```python
from build123d import *

# Parameters (mm, degrees)
SKETCH_1_W      = 20
SKETCH_1_H      = 13.2
SKETCH_1_R      = 1
EXTRUDE_1_DEPTH = 1.3
SKETCH_1_3_W    = 3.8
SKETCH_1_3_H    = 4.7
EXTRUDE_2_DEPTH = 3
SKETCH_1_4_W    = 1.6
SKETCH_1_4_H    = 0.7
EXTRUDE_3_DEPTH = 2.2
SKETCH_1_5_W    = 3.5
SKETCH_1_5_H    = 3
EXTRUDE_4_DEPTH = 3.5


with BuildPart() as part:
    # Sketch 1 → Extrude 1 (new body)
    with BuildSketch(Plane(origin=(0, 0, 0), x_dir=(1, 0, 0), z_dir=(0, 1, 0))):
        Rectangle(SKETCH_1_W, SKETCH_1_H)
        with Locations(Location((8.6, 5.2, 0), (0, 0, 270))):
            Circle(SKETCH_1_R, mode=Mode.SUBTRACT)
        with Locations(Location((-8.6, -5.2, 0), (0, 0, 270))):
            Circle(SKETCH_1_R, mode=Mode.SUBTRACT)
    extrude(amount=EXTRUDE_1_DEPTH)

    # Sketch 1_3 → Extrude 2 (add)
    with BuildSketch(Plane(origin=(0, 0, 0), x_dir=(1, 0, 0), z_dir=(0, 1, 0))):
        with Locations((-3.1, 3.25)):
            Rectangle(SKETCH_1_3_W, SKETCH_1_3_H)
        with Locations((-3.1, -3.25)):
            Rectangle(SKETCH_1_3_W, SKETCH_1_3_H)
    extrude(amount=EXTRUDE_2_DEPTH)

    # Sketch 1_4 → Extrude 3 (add)
    with BuildSketch(Plane(origin=(0, 0, 0), x_dir=(1, 0, 0), z_dir=(0, 1, 0))):
        with Locations((3.1, 4.65)):
            Rectangle(SKETCH_1_4_W, SKETCH_1_4_H)
        with Locations((3.1, 2.45)):
            Rectangle(SKETCH_1_4_W, SKETCH_1_4_H)
        with Locations((3.1, 0.25)):
            Rectangle(SKETCH_1_4_W, SKETCH_1_4_H)
    extrude(amount=EXTRUDE_3_DEPTH)

    # Sketch 1_5 → Extrude 4 (add)
    with BuildSketch(Plane(origin=(0, 0, 0), x_dir=(1, 0, 0), z_dir=(0, 1, 0))):
        with Locations((4.05, -3.1)):
            Rectangle(SKETCH_1_5_W, SKETCH_1_5_H)
    extrude(amount=EXTRUDE_4_DEPTH)


solid = part.part
```
Check sheet for the modelled part. Datum: model origin and axes. Units: mm. A direction names the side the tool comes from. Round coordinates to 2 decimals unless told otherwise and drop trailing zeros. Write each loop counter-clockwise with the first axis right and the second up, starting at its lowest first coordinate (ties: lowest second). Pieces come first, ordered by that corner, then holes. Notation, with made-up numbers: M 7.5,-3 L 59.5,-3 A19 ccw 59.5,27 Z; hole C 0.25,53.5 d2. An arc over 180 degrees is marked long. Write item = value, one per line. Start each with the question number.
1. Section check B-B, the plane z = 5.2. Record the cut outline in (x, y), then the cut area to 3 significant figures.
2. Scan lines: line 1 (Z direction, x = -4.25, y = 2.45); line 2 (X direction, y = 0.4, z = -5.2); line 3 (Y direction, x = 8, z = 2.25). Record each from-to range of solid material in increasing order. Write a range as [from, to].
3. Gauge pin test, flat ends, axial feed: pin 1 (1.9 mm diameter, centred on y = 2.5, z = 2, fed in from -X); pin 2 (1.5 mm diameter, centred on x = 1.5, z = 2.5, fed in from +Y); pin 3 (1.8 mm diameter, centred on x = 4, y = 2.5, fed in from -Z). Record the tip position at first contact, or that the pin passes through.
4. Section check C-C, the plane x = -2. Record the cut outline in (y, z), then the cut area to 3 significant figures.
5. Tool access check on faces 4 (the flat face through (-3, 2, 0.9)), 5 (the flat face through (-3, 2, 5.6)), 6 (the flat face through (-1.2, 2, -3)), 7 (the flat face through (3, 2, -4.3)), 8 (the flat face through (-5, 2, 3)). Record the directions out of +Z, -Z, +X, -X, +Y, -Y that give a thin tool (end or side, any length) a straight path to the whole face; none if there is none.
6. Section check D-D, the plane z = -3. Record the cut outline in (x, y), then the cut area to 3 significant figures.
7. Section check A-A, the plane x = -8.6. Record the cut outline in (y, z), then the cut area to 3 significant figures.
8. Release check for a two-part mould opening along X. For faces 1 (the flat face through (-10, 1, 0)), 2 (the flat face through (2.3, 2, 3)), 3 (the flat face through (3, 2, -2.8)) record: pulls with the +X half, pulls with the -X half, needs draft (parallel to the pull), parting line crosses it, or undercut.
Results found:
q1.outline = M -10,0 L -9.6,0 L -9.6,1.3 L -10,1.3 Z; M -7.6,0 L 10,0 L 10,1.3 L -1.2,1.3 L -1.2,3 L -5,3 L -5,1.3 L -7.6,1.3 Z
q1.area = 29.9 mm^2
q2.line_1 = [-5.6, -0.9], [0.9, 5.6]
q2.line_2 = [-10, 7.6], [9.6, 10]
q2.line_3 = [0, 1.3]
q3.pin_1 = -5
q3.pin_2 = 1.3
q3.pin_3 = -5
q4.outline = M 0,-6.6 L 1.3,-6.6 L 1.3,-5.6 L 3,-5.6 L 3,-0.9 L 1.3,-0.9 L 1.3,0.9 L 3,0.9 L 3,5.6 L 1.3,5.6 L 1.3,6.6 L 0,6.6 Z
q4.area = 33.1 mm^2
q5.face_4 = +X, -X, +Y
q5.face_5 = +Z, +X, -X, +Y
q5.face_6 = +Z, -Z, +Y
q5.face_7 = +X, +Y
q5.face_8 = +Z, -Z, -X, +Y
q6.outline = M -10,0 L 10,0 L 10,1.3 L -1.2,1.3 L -1.2,3 L -5,3 L -5,1.3 L -10,1.3 Z
q6.area = 32.5 mm^2
q7.outline = M 0,-6.6 L 1.3,-6.6 L 1.3,4.2 L 0,4.2 Z; M 0,6.2 L 1.3,6.2 L 1.3,6.6 L 0,6.6 Z
q7.area = 14.6 mm^2
q8.face_1 = pulls with the -X half
q8.face_2 = undercut
q8.face_3 = needs draft
